Here's how the part is built. I have some questions about the finished solid (model axes, mm). Face numbers are marked on the shaded views. A direction names the side the tool comes from. Give positions to 0.01 mm unless a question says otherwise; leave off trailing zeros. Loops run counter-clockwise (first coordinate to the right, second up) from the corner with the lowest first, then second, coordinate; pieces in that order, holes last. Notation, with made-up numbers: (-36, 44.5) - (-14, 44.5) arc R26 cw to (-14, 62.5) - close; hole circle Ø2 at (65, -27.75). An arc over 180 degrees is marked (long way). Use one line per item in the form item = value.
from build123d import *

# Parameters (mm, degrees)
SKETCH2_W                = 10
SKETCH2_H                = 42.5
SKETCH2_R                = 1.15
BOSS_EXTRUDE1_DEPTH      = 5
BOSS_EXTRUDE2_DEPTH      = 4
BOSS_EXTRUDE2_DEPTH_BACK = 4
SKETCH4_R                = 2.65
CUT_EXTRUDE1_DEPTH       = 12
SKETCH5_W                = 4
SKETCH5_H                = 8
CUT_EXTRUDE2_DEPTH       = 51.122350304
FILLET1_R                = 2
FILLET2_R                = 1


# Some blends are built 0.0001 mm under size
with BuildPart() as part:
    # Sketch2 → Boss-Extrude1 (new body)
    with BuildSketch(Plane(origin=(0, 0, 0), x_dir=(1, 0, 0), z_dir=(0, 1, 0))):
        with Locations((5, -21.25)):
            Rectangle(SKETCH2_W, SKETCH2_H)
        with Locations(Location((5, -40, 0), (0, 0, 270))):
            Circle(SKETCH2_R, mode=Mode.SUBTRACT)
    extrude(amount=BOSS_EXTRUDE1_DEPTH)

    # Sketch3 → Boss-Extrude2 (add, two sides: drawn at the far end of the back side and taken through both)
    with BuildSketch(Plane(origin=(5, 0, 0), x_dir=(0, 0, -1), z_dir=(1, 0, 0)).offset(-BOSS_EXTRUDE2_DEPTH_BACK)):
        Polygon((0, 5), (-20, 5), (0, 25), align=None)
    extrude(amount=BOSS_EXTRUDE2_DEPTH + BOSS_EXTRUDE2_DEPTH_BACK)

    # Sketch4 → Cut-Extrude1 (cut)
    with BuildSketch(Plane(origin=(0, 0, 0), x_dir=(-1, 0, 0), z_dir=(0, 0, -1))):
        with Locations((-5, 10)):
            Circle(SKETCH4_R)
    extrude(amount=-CUT_EXTRUDE1_DEPTH, mode=Mode.SUBTRACT)

    # Sketch5 → Cut-Extrude2 (cut, through all)
    with BuildSketch(Plane(origin=(9, 0, 0), x_dir=(0, 0, -1), z_dir=(1, 0, 0))):
        with Locations((-7, 10)):
            Rectangle(SKETCH5_W, SKETCH5_H)
    extrude(amount=-CUT_EXTRUDE2_DEPTH, mode=Mode.SUBTRACT)

    # Fillet1
    # the kernel refuses this fillet: 2 mm, written as the material it adds along each edge
    with BuildSketch(Plane(origin=(1, 5, 0), x_dir=(-1, 0, 0), z_dir=(0, 0, 1))) as fillet1_piece_1_section:
        with BuildLine():
            CenterArc((2, -1.732050808), FILLET1_R, 120, 60)
            Line((0, -1.732050808), (0, 0))
            Line((0, 0), (1, 0))
        make_face()
    fillet1_piece_1 = extrude(amount=24.330127019, mode=Mode.PRIVATE)
    fillet1_piece_1 = split(fillet1_piece_1, bisect_by=Plane(origin=(1, 15, 10), z_dir=(0, -0.7071067811865475, -0.7071067811865476)), keep=Keep.TOP, mode=Mode.PRIVATE)
    fillet1_piece_1 = split(fillet1_piece_1, bisect_by=Plane(origin=(1, 6, 0), z_dir=(0, -1, 0)), keep=Keep.TOP, mode=Mode.PRIVATE)
    add(fillet1_piece_1)
    with BuildSketch(Plane(origin=(1, 5, 0), x_dir=(-1, 0, 0), z_dir=(0, 0, 1))) as fillet1_piece_2_section:
        with BuildLine():
            CenterArc((2, -1.732050808), FILLET1_R, 120, 60)
            Line((0, -1.732050808), (0, 0))
            Line((0, 0), (1, 0))
        make_face()
    fillet1_piece_2 = extrude(amount=24.330127019, mode=Mode.PRIVATE)
    fillet1_piece_2 = split(fillet1_piece_2, bisect_by=Plane(origin=(1, 5, 5), z_dir=(0, 0, -1)), keep=Keep.TOP, mode=Mode.PRIVATE)
    add(fillet1_piece_2)
    with BuildSketch(Plane(origin=(1, 5, -4.330127019), x_dir=(-1, 0, 0), z_dir=(0, 0, 1))) as fillet1_piece_3_section:
        with BuildLine():
            CenterArc((2, -1.732050808), FILLET1_R, 120, 60)
            Line((0, -1.732050808), (0, 0))
            Line((0, 0), (1, 0))
        make_face()
    fillet1_piece_3 = extrude(amount=28.660254038, mode=Mode.PRIVATE)
    fillet1_piece_3 = split(fillet1_piece_3, bisect_by=Plane(origin=(1, 17.165063509, 7.834936491), z_dir=(0, -0.7071067811865475, -0.7071067811865476)), keep=Keep.TOP, mode=Mode.PRIVATE)
    fillet1_piece_3 = split(fillet1_piece_3, bisect_by=Plane(origin=(1, 5, 9), z_dir=(0, 0, 1)), keep=Keep.TOP, mode=Mode.PRIVATE)
    add(fillet1_piece_3)
    with BuildSketch(Plane(origin=(9, 5, 0), x_dir=(1, 0, 0), z_dir=(0, 0, 1))) as fillet1_piece_4_section:
        with BuildLine():
            CenterArc((2, 1.732050808), FILLET1_R, 180, 60)
            Line((0, 1.732050808), (0, 0))
            Line((0, 0), (1, 0))
        make_face()
    fillet1_piece_4 = extrude(amount=24.330127019, mode=Mode.PRIVATE)
    fillet1_piece_4 = split(fillet1_piece_4, bisect_by=Plane(origin=(9, 15, 10), z_dir=(0, -0.7071067811865475, -0.7071067811865476)), keep=Keep.TOP, mode=Mode.PRIVATE)
    fillet1_piece_4 = split(fillet1_piece_4, bisect_by=Plane(origin=(9, 6, 0), z_dir=(0, -1, 0)), keep=Keep.TOP, mode=Mode.PRIVATE)
    add(fillet1_piece_4)
    with BuildSketch(Plane(origin=(9, 5, 0), x_dir=(1, 0, 0), z_dir=(0, 0, 1))) as fillet1_piece_5_section:
        with BuildLine():
            CenterArc((2, 1.732050808), FILLET1_R, 180, 60)
            Line((0, 1.732050808), (0, 0))
            Line((0, 0), (1, 0))
        make_face()
    fillet1_piece_5 = extrude(amount=24.330127019, mode=Mode.PRIVATE)
    fillet1_piece_5 = split(fillet1_piece_5, bisect_by=Plane(origin=(9, 5, 5), z_dir=(0, 0, -1)), keep=Keep.TOP, mode=Mode.PRIVATE)
    add(fillet1_piece_5)
    with BuildSketch(Plane(origin=(9, 5, -4.330127019), x_dir=(1, 0, 0), z_dir=(0, 0, 1))) as fillet1_piece_6_section:
        with BuildLine():
            CenterArc((2, 1.732050808), FILLET1_R, 180, 60)
            Line((0, 1.732050808), (0, 0))
            Line((0, 0), (1, 0))
        make_face()
    fillet1_piece_6 = extrude(amount=28.660254038, mode=Mode.PRIVATE)
    fillet1_piece_6 = split(fillet1_piece_6, bisect_by=Plane(origin=(9, 17.165063509, 7.834936491), z_dir=(0, -0.7071067811865475, -0.7071067811865476)), keep=Keep.TOP, mode=Mode.PRIVATE)
    fillet1_piece_6 = split(fillet1_piece_6, bisect_by=Plane(origin=(9, 5, 9), z_dir=(0, 0, 1)), keep=Keep.TOP, mode=Mode.PRIVATE)
    add(fillet1_piece_6)
    with BuildSketch(Plane(origin=(9, 5, 20), x_dir=(0, 0, 1), z_dir=(-1, 0, 0))) as fillet1_piece_7:
        with BuildLine():
            CenterArc((FILLET1_R * 0.414213562373, FILLET1_R), FILLET1_R, 225, 45)
            Line((-FILLET1_R * 0.292893218813, FILLET1_R * 0.292893218813), (0, 0))
            Line((0, 0), (FILLET1_R * 0.414213562373, 0))
        make_face()
    extrude(amount=8)
    with BuildSketch(Plane(origin=(9, 5, 20), x_dir=(0, 0, 1), z_dir=(-1, 0, 0))) as fillet1_piece_8a_section:
        with BuildLine():
            CenterArc((FILLET1_R * 0.414213562373, FILLET1_R), FILLET1_R, 225, 45)
            Line((-FILLET1_R * 0.292893218813, FILLET1_R * 0.292893218813), (0, 0))
            Line((0, 0), (FILLET1_R * 0.414213562373, 0))
        make_face()
    fillet1_piece_8a = extrude(amount=10.071067812, mode=Mode.PRIVATE)
    fillet1_piece_8a = split(fillet1_piece_8a, bisect_by=Plane(origin=(0, 5, 20), z_dir=(1, 0, 0)), keep=Keep.TOP, mode=Mode.PRIVATE)
    fillet1_piece_8a = split(fillet1_piece_8a, bisect_by=Plane(origin=(1, 5, 20), z_dir=(-1, 0, 0)), keep=Keep.TOP, mode=Mode.PRIVATE)
    with BuildSketch(Plane(origin=(1, 5, 0), x_dir=(-1, 0, 0), z_dir=(0, 0, 1))) as fillet1_piece_8b_section:
        with BuildLine():
            CenterArc((2, -1.732050808), FILLET1_R, 120, 60)
            Line((0, -1.732050808), (0, 0))
            Line((0, 0), (1, 0))
        make_face()
    fillet1_piece_8b = extrude(amount=24.330127019, mode=Mode.PRIVATE)
    fillet1_piece_8b = split(fillet1_piece_8b, bisect_by=Plane(origin=(1, 15, 10), z_dir=(0, 0.7071067811865475, 0.7071067811865476)), keep=Keep.TOP, mode=Mode.PRIVATE)
    fillet1_piece_8b = split(fillet1_piece_8b, bisect_by=Plane(origin=(1, 6, 0), z_dir=(0, -1, 0)), keep=Keep.TOP, mode=Mode.PRIVATE)
    fillet1_piece_8 = fillet1_piece_8a & fillet1_piece_8b
    add(fillet1_piece_8)
    with BuildSketch(Plane(origin=(9, 5, 0), x_dir=(1, 0, 0), z_dir=(0, 0, 1))) as fillet1_piece_9a_section:
        with BuildLine():
            CenterArc((2, 1.732050808), FILLET1_R, 180, 60)
            Line((0, 1.732050808), (0, 0))
            Line((0, 0), (1, 0))
        make_face()
    fillet1_piece_9a = extrude(amount=24.330127019, mode=Mode.PRIVATE)
    fillet1_piece_9a = split(fillet1_piece_9a, bisect_by=Plane(origin=(9, 15, 10), z_dir=(0, 0.7071067811865475, 0.7071067811865476)), keep=Keep.TOP, mode=Mode.PRIVATE)
    fillet1_piece_9a = split(fillet1_piece_9a, bisect_by=Plane(origin=(9, 6, 0), z_dir=(0, -1, 0)), keep=Keep.TOP, mode=Mode.PRIVATE)
    with BuildSketch(Plane(origin=(11.071067812, 5, 20), x_dir=(0, 0, 1), z_dir=(-1, 0, 0))) as fillet1_piece_9b_section:
        with BuildLine():
            CenterArc((FILLET1_R * 0.414213562373, FILLET1_R), FILLET1_R, 225, 45)
            Line((-FILLET1_R * 0.292893218813, FILLET1_R * 0.292893218813), (0, 0))
            Line((0, 0), (FILLET1_R * 0.414213562373, 0))
        make_face()
    fillet1_piece_9b = extrude(amount=10.071067812, mode=Mode.PRIVATE)
    fillet1_piece_9b = split(fillet1_piece_9b, bisect_by=Plane(origin=(10, 5, 20), z_dir=(-1, 0, 0)), keep=Keep.TOP, mode=Mode.PRIVATE)
    fillet1_piece_9b = split(fillet1_piece_9b, bisect_by=Plane(origin=(9, 5, 20), z_dir=(1, 0, 0)), keep=Keep.TOP, mode=Mode.PRIVATE)
    fillet1_piece_9 = fillet1_piece_9a & fillet1_piece_9b
    add(fillet1_piece_9)
    # the kernel refuses this fillet: 2 mm, written as the material it takes off along each edge
    with BuildSketch(Plane(origin=(0, -5, 42.5), x_dir=(1, 0, 0), z_dir=(0, 1, 0))) as fillet1_2_piece_1:
        with BuildLine():
            CenterArc((FILLET1_R, FILLET1_R), FILLET1_R, 180, 90)
            Line((0, FILLET1_R), (0, 0))
            Line((0, 0), (FILLET1_R, 0))
        make_face()
    extrude(amount=15, mode=Mode.SUBTRACT)
    with BuildSketch(Plane(origin=(10, -5, 42.5), x_dir=(-1, 0, 0), z_dir=(0, 1, 0))) as fillet1_2_piece_2:
        with BuildLine():
            CenterArc((FILLET1_R, -FILLET1_R), FILLET1_R, 90, 90)
            Line((0, -FILLET1_R), (0, 0))
            Line((0, 0), (FILLET1_R, 0))
        make_face()
    extrude(amount=15, mode=Mode.SUBTRACT)

    # Fillet2
    fillet2_edges = [part.edges().sort_by_distance(p)[0] for p in [
        (0, 2.5, 0),
        (10, 2.5, 0),
        (5, 25, 0),
    ]]
    fillet(fillet2_edges, radius=FILLET2_R - 0.0001)  # a hair under: the kernel refuses the full size


solid = part.part
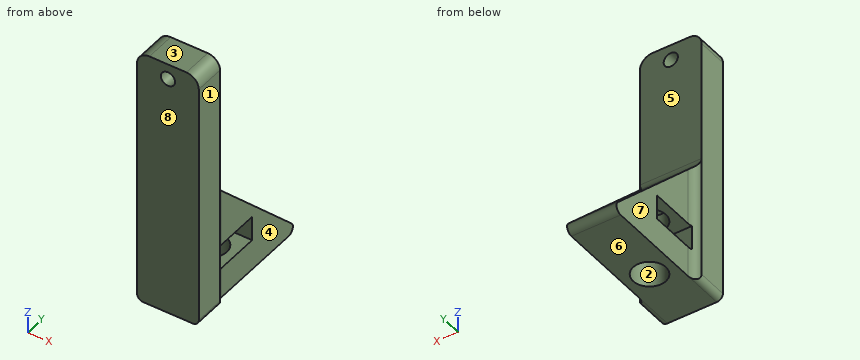
(1) Thinking about a two-plate mould opening in X: for the marked faces 1, 2 and 3, which applies, pulls with the +X half, pulls with the -X half, needs draft (parallel to the pull), parting line crosses it, or undercut?
Geometry says:
face_1 = pulls with the +X half
face_2 = undercut
face_3 = needs draft
(2) If we section it at A-A (x = 5): List the corners of the cut face in (y, z) for me, plus the area to 3 significant figures.
Geometry says:
outline = (0, 0) - (7.35, 0) - (7.35, 5) - (6, 5) - (6, 9) - (7.35, 9) - (7.35, 12) - (12.65, 12) - (12.65, 9) - (14, 9) - (14, 5) - (12.65, 5) - (12.65, 0) - (22.59, 0) arc R1 ccw to (23.29, 1.71) - (5.59, 19.41) arc R2 cw to (5, 20.83) - (5, 38.85) - (0, 38.85) - close; (0, 41.15) - (5, 41.15) - (5, 42.5) - (0, 42.5) - close
area = 325 mm²
(3) For the marked faces 4, 5, 6, 7 and 8, which set-ups out of +Z, -Z, +X, -X, +Y, -Y let a thin tool reach every point of the face, with its end or its side?
Geometry says:
face_4 = +Z, -Z, +X, +Y
face_5 = +Z, +X, -X, +Y
face_6 = -Z, +X, -X, +Y, -Y
face_7 = +Z, -Z, -X, +Y
face_8 = +Z, -Z, +X, -X, -Y
(4) For P1, Ø3, axis at x = 2, z = 5, coming from the +Y side; P2, Ø6, axis at x = 7, z = 6, coming from the -Y side; P3, Ø4.5, axis at x = 3.5, z = 6.5, coming from the +Y side; P4, Ø13.5, axis at y = 19, z = 8, coming from the -X side, each with a flat end and sliding along its axis, tell me the tip position at first contact or that it passes through.
Geometry says:
P1 = 21.5
P2 = 0
P3 = 20.75
P4 = 1
(5) If I drill on probe 1 along X at (y, z) = (3.9, 40); probe 2 along Y at (x, z) = (2.75, 7); probe 3 along Y at (x, z) = (5, 11.1), over which ranges is the centre line in solid material (lowest first)?
Geometry says:
probe_1 = 0 to 3.85, 6.15 to 10
probe_2 = 0 to 6, 14 to 18
probe_3 = 0 to 7.35, 12.65 to 13.9
(6) If we section it at B-B (z = 40): List the corners of the cut face in (x, y) for me.
Geometry says:
outline = (0, 0) - (3.85, 0) - (3.85, 5) - (0, 5) - close; (6.15, 0) - (10, 0) - (10, 5) - (6.15, 5) - close
(7) If we section it at D-D (z = 14.5): List the corners of the cut face in (x, y) for me, plus the area to 3 significant figures.
Geometry says:
outline = (0, 0) - (10, 0) - (10, 5) arc R2 cw to (9, 6.73) - (9, 10.5) - (1, 10.5) - (1, 6.73) arc R2 cw to (0, 5) - close
area = 95.0 mm²
(8) If we section it at C-C (y = 8.75): List the corners of the cut face in (x, z) for me, plus the area to 3 significant figures.
Geometry says:
outline = (1, 0) - (2.66, 0) - (2.66, 5) - (1, 5) - close; (1, 9) - (2.66, 9) - (2.66, 12) - (7.34, 12) - (7.34, 9) - (9, 9) - (9, 16.25) - (1, 16.25) - close; (7.34, 0) - (9, 0) - (9, 5) - (7.34, 5) - close
area = 60.6 mm²
